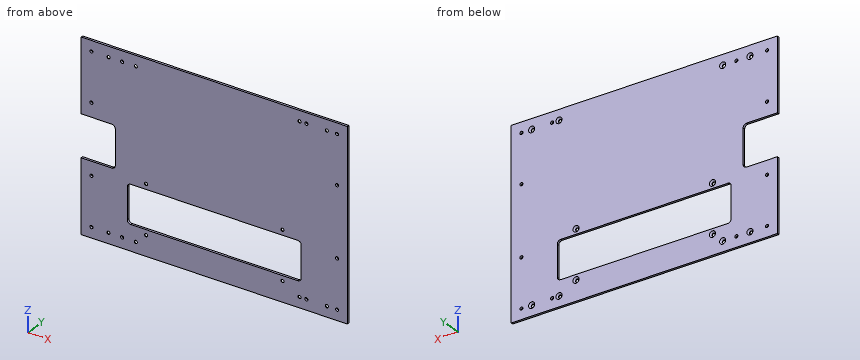
```python
from build123d import *

# Parameters (mm, degrees)
SKETCH1_W                            = 390
SKETCH1_H                            = 270
BOSS_EXTRUDE1_DEPTH                  = 3.175
CSK_FOR_M4_SFHCS2_AT_2_COUNT         = 2
CSK_FOR_M4_SFHCS2_AT_2_PITCH         = 40
CSK_FOR_M4_SFHCS2_AT_3_COUNT         = 2
CSK_FOR_M4_SFHCS2_AT_3_PITCH         = 280
CSK_FOR_M4_SFHCS2_AT_4_COUNT         = 2
CSK_FOR_M4_SFHCS2_AT_4_PITCH         = 320
M4_CLEARANCE_HOLE1_D                 = 4.5
MIRROR3_AT_THE_SECOND_PLANE_COPY_1_D = 4.5
SKETCH10_W                           = 255
SKETCH10_H                           = 55
CUT_EXTRUDE1_DEPTH                   = 3.175
SKETCH11_W                           = 50
SKETCH11_H                           = 60
CUT_EXTRUDE2_DEPTH                   = 10
CSK_FOR_M4_SFHCS3_AT_2_COUNT         = 2
CSK_FOR_M4_SFHCS3_AT_2_PITCH         = 211.896201004
CSK_FOR_M4_SFHCS3_AT_3_COUNT         = 2
CSK_FOR_M4_SFHCS3_AT_3_PITCH         = 200
CSK_FOR_M4_SFHCS3_AT_4_COUNT         = 2
CSK_FOR_M4_SFHCS3_AT_4_PITCH         = 70
FILLET1_R                            = 5
FILLET2_R                            = 5


with BuildPart() as part:
    # Sketch1 → Boss-Extrude1 (new body)
    with BuildSketch(Plane(origin=(0, 0, 0), x_dir=(1, 0, 0), z_dir=(0, 1, 0))):
        Rectangle(SKETCH1_W, SKETCH1_H)
    extrude(amount=BOSS_EXTRUDE1_DEPTH)

    # Sketch6 → CSK for M4 SFHCS2 (revolve, cut)
    with BuildSketch(Plane(origin=(-155, 3.175, -120), x_dir=(0, 0, 1), z_dir=(1, 0, 0))):
        Polygon((0, 0), (0, 3.175), (2.25, 3.175), (2.25, 2.23), (4.48, 0), align=None)
    csk_for_m4_sfhcs2 = revolve(axis=Axis((-155, 9.525, -120), (0, -1, 0)), mode=Mode.SUBTRACT)

    # CSK for M4 SFHCS2 at 2: CSK for M4 SFHCS2 ×2
    with Locations(*[(i * CSK_FOR_M4_SFHCS2_AT_2_PITCH, 0, 0) for i in range(1, CSK_FOR_M4_SFHCS2_AT_2_COUNT)]):
        add(csk_for_m4_sfhcs2, mode=Mode.SUBTRACT)

    # CSK for M4 SFHCS2 at 3: CSK for M4 SFHCS2 ×2
    with Locations(*[(i * CSK_FOR_M4_SFHCS2_AT_3_PITCH, 0, 0) for i in range(1, CSK_FOR_M4_SFHCS2_AT_3_COUNT)]):
        add(csk_for_m4_sfhcs2, mode=Mode.SUBTRACT)

    # CSK for M4 SFHCS2 at 4: CSK for M4 SFHCS2 ×2
    with Locations(*[(i * CSK_FOR_M4_SFHCS2_AT_4_PITCH, 0, 0) for i in range(1, CSK_FOR_M4_SFHCS2_AT_4_COUNT)]):
        add(csk_for_m4_sfhcs2, mode=Mode.SUBTRACT)

    # Mirror2: CSK for M4 SFHCS2 across plane
    add(csk_for_m4_sfhcs2.mirror(Plane.XY), mode=Mode.SUBTRACT)

    # Mirror2 copy 1 sketch → Mirror2 copy 1 (revolve, cut)
    with BuildSketch(Plane(origin=(-115, 3.175, 120), x_dir=(0, 0, -1), z_dir=(1, 0, 0))):
        Polygon((0, 0), (0, -3.175), (2.25, -3.175), (2.25, -2.23), (4.48, 0), align=None)
    revolve(axis=Axis((-115, 9.525, 120), (0, 1, 0)), mode=Mode.SUBTRACT)

    # Mirror2 copy 2 sketch → Mirror2 copy 2 (revolve, cut)
    with BuildSketch(Plane(origin=(125, 3.175, 120), x_dir=(0, 0, -1), z_dir=(1, 0, 0))):
        Polygon((0, 0), (0, -3.175), (2.25, -3.175), (2.25, -2.23), (4.48, 0), align=None)
    revolve(axis=Axis((125, 9.525, 120), (0, 1, 0)), mode=Mode.SUBTRACT)

    # Mirror2 copy 3 sketch → Mirror2 copy 3 (revolve, cut)
    with BuildSketch(Plane(origin=(165, 3.175, 120), x_dir=(0, 0, -1), z_dir=(1, 0, 0))):
        Polygon((0, 0), (0, -3.175), (2.25, -3.175), (2.25, -2.23), (4.48, 0), align=None)
    revolve(axis=Axis((165, 9.525, 120), (0, 1, 0)), mode=Mode.SUBTRACT)

    # M4 Clearance Hole1 (through all)
    with Locations(Plane(origin=(0, 3.175, 0), x_dir=(1, 0, 0), z_dir=(0, 1, 0))):
        with Locations((-180, 120), (-180, 50), (-135, 120)):
            m4_clearance_hole1 = Hole(M4_CLEARANCE_HOLE1_D / 2)

    # Mirror3: M4 Clearance Hole1 across plane
    add(m4_clearance_hole1.mirror(Plane(origin=(0, 0, 0), x_dir=(0, 0, 1), z_dir=(1, 0, 0))), mode=Mode.SUBTRACT)

    # Mirror3 at the second plane: M4 Clearance Hole1 across plane
    add(m4_clearance_hole1.mirror(Plane.XY), mode=Mode.SUBTRACT)

    # Mirror3 at the second plane copy 1 (through all)
    with Locations(Plane(origin=(0, 3.175, 0), x_dir=(-1, 0, 0), z_dir=(0, 1, 0))):
        with Locations((-180, 120), (-180, 50), (-135, 120)):
            Hole(MIRROR3_AT_THE_SECOND_PLANE_COPY_1_D / 2)

    # Sketch10 → Cut-Extrude1 (cut)
    with BuildSketch(Plane(origin=(0, 3.175, 0), x_dir=(1, 0, 0), z_dir=(0, 1, 0))):
        with Locations((0, 71)):
            Rectangle(SKETCH10_W, SKETCH10_H)
    extrude(amount=-CUT_EXTRUDE1_DEPTH, mode=Mode.SUBTRACT)

    # Sketch11 → Cut-Extrude2 (cut)
    with BuildSketch(Plane(origin=(0, 3.175, 0), x_dir=(1, 0, 0), z_dir=(0, 1, 0))):
        with Locations((-170, 0)):
            Rectangle(SKETCH11_W, SKETCH11_H)
    extrude(amount=-CUT_EXTRUDE2_DEPTH, mode=Mode.SUBTRACT)

    # Sketch13 → CSK for M4 SFHCS3 (revolve, cut)
    with BuildSketch(Plane(origin=(100, 3.175, -106), x_dir=(0, 0, 1), z_dir=(1, 0, 0))):
        Polygon((0, 0), (0, 3.175), (2.25, 3.175), (2.25, 2.23), (4.48, 0), align=None)
    csk_for_m4_sfhcs3 = revolve(axis=Axis((100, 9.525, -106), (0, -1, 0)), mode=Mode.SUBTRACT)

    # CSK for M4 SFHCS3 at 2: CSK for M4 SFHCS3 ×2
    with Locations(*[Vector(-0.9438583563660174, 0, 0.33035042472810616) * (i * CSK_FOR_M4_SFHCS3_AT_2_PITCH) for i in range(1, CSK_FOR_M4_SFHCS3_AT_2_COUNT)]):
        add(csk_for_m4_sfhcs3, mode=Mode.SUBTRACT)

    # CSK for M4 SFHCS3 at 3: CSK for M4 SFHCS3 ×2
    with Locations(*[(-i * CSK_FOR_M4_SFHCS3_AT_3_PITCH, 0, 0) for i in range(1, CSK_FOR_M4_SFHCS3_AT_3_COUNT)]):
        add(csk_for_m4_sfhcs3, mode=Mode.SUBTRACT)

    # CSK for M4 SFHCS3 at 4: CSK for M4 SFHCS3 ×2
    with Locations(*[(0, 0, i * CSK_FOR_M4_SFHCS3_AT_4_PITCH) for i in range(1, CSK_FOR_M4_SFHCS3_AT_4_COUNT)]):
        add(csk_for_m4_sfhcs3, mode=Mode.SUBTRACT)

    # Fillet1
    fillet1_edges = [part.edges().sort_by_distance(p)[0] for p in [
        (127.5, 1.5875, -98.5),
        (127.5, 1.5875, -43.5),
        (-127.5, 1.5875, -43.5),
        (-127.5, 1.5875, -98.5),
    ]]
    fillet(fillet1_edges, radius=FILLET1_R)

    # Fillet2
    fillet2_edges = [part.edges().sort_by_distance(p)[0] for p in [
        (-145, 1.5875, -30),
        (-145, 1.5875, 30),
    ]]
    fillet(fillet2_edges, radius=FILLET2_R)


solid = part.part
```
Check sheet for the modelled part. Datum: model origin and axes. Units: mm. Round coordinates to 2 decimals unless told otherwise and drop trailing zeros. Loops run counter-clockwise (first coordinate to the right, second up) from the corner with the lowest first, then second, coordinate; pieces in that order, holes last. Notation, with made-up numbers: (15.5, -1) - (34.5, -1) arc R22 cw to (34.5, 10) - close; hole circle Ø6 at (12.25, 79). An arc over 180 degrees is marked (long way). Answer as a JSON object with one key per item and string values. Group by question number.
Q1. Gauge pin test, flat end, axial feed: P1, Ø1, axis at y = 1.5, z = -6.5, coming from the -X side. Record the tip position at first contact, or that the pin passes through.
Q2. Scan lines: line 1 along Z through (x, y) = (-135, 2.25); line 2 along X through (y, z) = (0.25, -106); line 3 along Z through (x, y) = (180, 1.45). Record each from-to range of solid material in increasing order. Write a range as [from, to].
Q3. Sectioned sample at A-A, the plane z = -76. Enter the section's corners in (x, y) (3 decimals), plus the area to 3 significant figures.
Q4. Sectioned sample at C-C, the plane z = 18.5. Enter the section's corners in (x, y) (3 decimals).
Q5. Sectioned sample at D-D, the plane y = 1.6. Count the separate pieces of the cut face and the enclosed holes in it, plus the area to 3 significant figures.
Q6. Sectioned sample at B-B, the plane x = 35. Enter the section's corners in (y, z) (3 decimals).
Solution:
{
 "1": {"P1": "stops at x = -145"},
 "2": {"line 1": "z = [-135, -122.25], [-117.75, 117.75], [122.25, 135]", "line 2": "x = [-195, -102.25], [-97.75, 97.75], [102.25, 195]", "line 3": "z = [-135, -122.25], [-117.75, -52.25], [-47.75, 47.75], [52.25, 117.75], [122.25, 135]"},
 "3": {"outline": "(-195, 0) - (-127.5, 0) - (-127.5, 3.175) - (-195, 3.175) - close; (127.5, 0) - (195, 0) - (195, 3.175) - (127.5, 3.175) - close", "area": "429 mm²"},
 "4": {"outline": "(-145, 0) - (195, 0) - (195, 3.175) - (-145, 3.175) - close"},
 "5": {"separate pieces": "1", "enclosed holes": "25", "area": "87,800 mm²"},
 "6": {"outline": "(0, -135) - (3.175, -135) - (3.175, -98.5) - (0, -98.5) - close; (0, -43.5) - (3.175, -43.5) - (3.175, 135) - (0, 135) - close"}
}
